Geometry check sheet. Reference: the model listing, model coordinates, mm. A direction names the side the tool comes from. Round coordinates to 2 decimals unless told otherwise and drop trailing zeros. Loops run counter-clockwise (first coordinate to the right, second up) from the corner with the lowest first, then second, coordinate; pieces in that order, holes last. Notation, with made-up numbers: M 32,33.5 L 44,33.5 A23 ccw 44,53.5 Z; hole C 27,57 d8. An arc over 180 degrees is marked long. Use one line per item in the form item = value. Start each with the question number.
1. Cross-section at A-A (z = 19.5). Record the boundary of the cut face in (x, y), then the cut area to 3 significant figures.
2. Cross-section at B-B (x = 0). Record the boundary of the cut face in (y, z), then the cut area to 4 significant figures.
3. Cross-section at C-C (y = 13). Record the boundary of the cut face in (x, z), then the cut area to 3 significant figures.
4. Draft check along X on faces 1 (the flat face through (20, 0, 3)), 2 (the flat face through (0, 20, 3)), 3 (the cylindrical face through (-16.5, 13.07, 3.55)), 4 (the flat face through (-10, -2, 19)). Enter one of: pulls with the +X half, pulls with the -X half, needs draft (parallel to the pull), parting line crosses it, or undercut.
5. Cross-section at D-D (x = 15). Record the boundary of the cut face in (y, z), then the cut area to 3 significant figures.
6. Go/stop test with flat-tipped pins: pin 1 (16 mm diameter, centred on x = -2.5, z = 16.5, fed in from +Y); pin 2 (1.8 mm diameter, centred on x = 15, y = 13, fed in from +Z); pin 3 (0.9 mm diameter, centred on y = -2, z = 25.5, fed in from -X); pin 4 (4 mm diameter, centred on x = -3, z = 11.5, fed in from -Y). Record where each tip stops, or that it passes through.
7. Set-up check for faces 5 (the flat face through (10, -2, 19)), 6 (the flat face through (0, 0, 0)), 7 (the flat face through (-5, 0, 19)), 8 (the flat face through (-5, -3, 19)), 9 (the flat face through (0, -1, 32)): record each of +Z, -Z, +X, -X, +Y, -Y from which the full face is reachable in a straight line by a thin tool's end or side.
8. Material ranges on line 1 (Y direction, x = -15, z = 2.75); line 2 (X direction, y = -1.65, z = 19.5); line 3 (Z direction, x = 2, y = 13), recorded low to high.
```python
from build123d import *

# Parameters (mm, degrees)
F0_W     = 40
F0_H     = 40
F1_DEPTH = 7
F3_W     = 20
F3_H     = 3
F4_DEPTH = 25
F5_R     = 1.5
F6_DEPTH = 25
F7_R     = 4.25
F8_DEPTH = 25


with BuildPart() as f1:
    # F0 (on Top) → F1 (new body)
    with BuildSketch(Plane.XY):
        Rectangle(F0_W, F0_H)
    extrude(amount=F1_DEPTH)

    # F3 (on offset) → F4 (join)
    with BuildSketch(Plane.XY.offset(7)):
        with Locations((0, -1.5)):
            Rectangle(F3_W, F3_H)
    extrude(amount=F4_DEPTH)

    # F5 (on offset) → F6 (cut)
    with BuildSketch(Plane.XY.offset(7)):
        with Locations((-15, 13)):
            Circle(F5_R)
        with Locations((15, 13)):
            Circle(F5_R)
    extrude(amount=-F6_DEPTH, mode=Mode.SUBTRACT)

    # F7 (on Front) → F8 (cut)
    with BuildSketch(Plane.XZ):
        with Locations((0, 19.5)):
            Circle(F7_R)
    extrude(amount=F8_DEPTH, mode=Mode.SUBTRACT)


solid = f1.part
```
Reported:
q1.outline = M -10,-3 L -4.25,-3 L -4.25,0 L -10,0 Z; M 4.25,-3 L 10,-3 L 10,0 L 4.25,0 Z
q1.area = 34.5 mm²
q2.outline = M -20,0 L 20,0 L 20,7 L 0,7 L 0,15.25 L -3,15.25 L -3,7 L -20,7 Z; M -3,23.75 L 0,23.75 L 0,32 L -3,32 Z
q2.area = 329.5 mm²
q3.outline = M -20,0 L -16.5,0 L -16.5,7 L -20,7 Z; M -13.5,0 L 13.5,0 L 13.5,7 L -13.5,7 Z; M 16.5,0 L 20,0 L 20,7 L 16.5,7 Z
q3.area = 238 mm²
q4.face_1 = pulls with the +X half
q4.face_2 = needs draft
q4.face_3 = undercut
q4.face_4 = pulls with the -X half
q5.outline = M -20,0 L 11.5,0 L 11.5,7 L -20,7 Z; M 14.5,0 L 20,0 L 20,7 L 14.5,7 Z
q5.area = 259 mm²
q6.pin_1 = 0
q6.pin_2 = through
q6.pin_3 = -10
q6.pin_4 = -3
q7.face_5 = +Z, +X, +Y, -Y
q7.face_6 = -Z, +X, -X, +Y, -Y
q7.face_7 = +Z, +X, -X, +Y
q7.face_8 = +Z, +X, -X, -Y
q7.face_9 = +Z, +X, -X, +Y, -Y
q8.line_1 = -20 to 11.5, 14.5 to 20
q8.line_2 = -10 to -4.25, 4.25 to 10
q8.line_3 = 0 to 7
